Job drawing, mm, ordinate dimensions from the low corner. One solid piece. Round coordinates to 2 decimals unless told otherwise and drop trailing zeros. Loops run counter-clockwise (first coordinate to the right, second up) from the corner with the lowest first, then second, coordinate; pieces in that order, holes last. Notation, with made-up numbers: M 12,-35.75 L 42,-35.75 A33 ccw 42,3.25 Z; hole C 53,-36 d9. An arc over 180 degrees is marked long. Use a Markdown table: item, result. Add a question column.
(1) Band-saw the part on C-C, the plane x = 18. Write the cut outline in (y, z), and give its area (3 significant figures).
(2) Flat gauge pins, fed straight in: P1, Ø1.5, axis at x = 12.5, z = 1.5, coming from the -Y side; P2, Ø6, axis at x = 19, y = 9.5, coming from the -Z side; P3, Ø1.5, axis at y = 15, z = 1, coming from the +X side. Where does each tip first touch, or does it go through?
(3) Band-saw the part on D-D, the plane z = 0.65. Write the cut outline in (x, y) (3 decimals).
(4) Band-saw the part on B-B, the plane x = 11.43. Write the cut outline in (y, z) (3 decimals).
(5) Wall check: L1, parallel to Y at x = 11.43, z = 1.85 (3 decimals); L2, parallel to X at y = 11.75, z = 1.5; L3, parallel to Y at x = 15.25, z = 0.35. Give the ranges that are in metal, low to high.
(6) Band-saw the part on A-A, the plane y = 11.43. Write the cut outline in (x, z) (3 decimals), and give its area (3 significant figures).
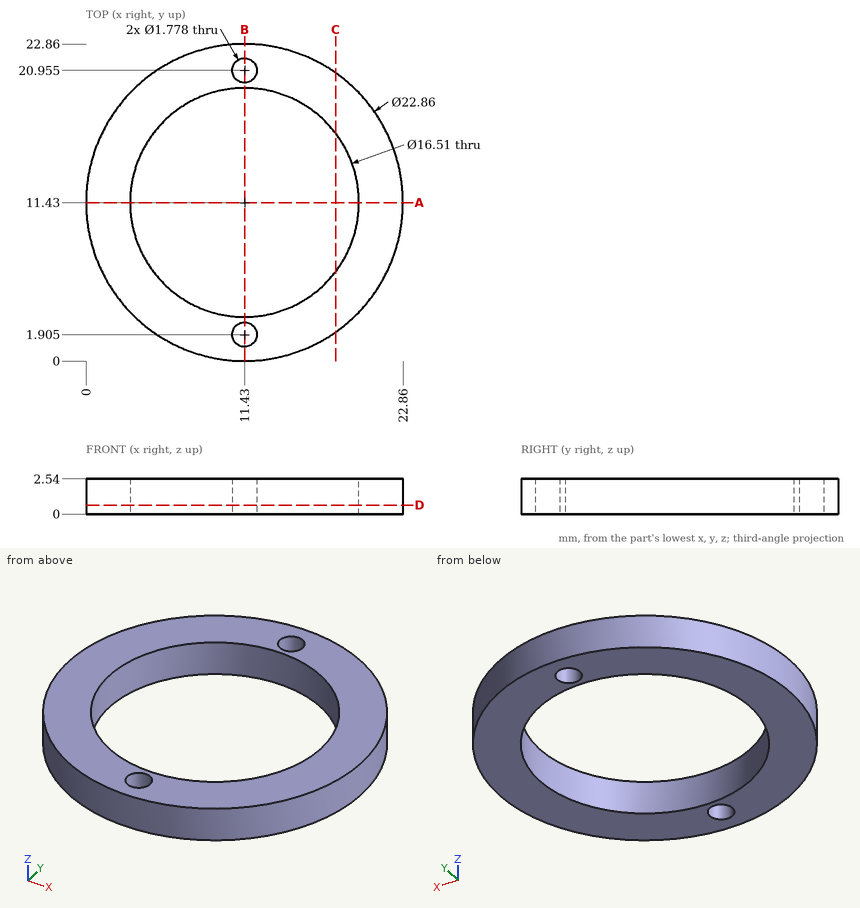
Return value:
| question | item | result |
|---|---|---|
| 1 | outline | M 2.08,0 L 6.43,0 L 6.43,2.54 L 2.08,2.54 Z; M 16.43,0 L 20.78,0 L 20.78,2.54 L 16.43,2.54 Z |
| 1 | area | 22.1 mm^2 |
| 2 | P1 | y = 0 |
| 2 | P2 | z = 0 |
| 2 | P3 | x = 22.51 |
| 3 | outline | C 11.43,11.43 d22.86; hole C 11.43,11.43 d16.51; hole C 11.43,1.905 d1.778; hole C 11.43,20.955 d1.778 |
| 4 | outline | M 0,0 L 1.016,0 L 1.016,2.54 L 0,2.54 Z; M 2.794,0 L 3.175,0 L 3.175,2.54 L 2.794,2.54 Z; M 19.685,0 L 20.066,0 L 20.066,2.54 L 19.685,2.54 Z; M 21.844,0 L 22.86,0 L 22.86,2.54 L 21.844,2.54 Z |
| 5 | L1 | 0 to 1.016, 2.794 to 3.175, 19.685 to 20.066, 21.844 to 22.86 |
| 5 | L2 | 0 to 3.18, 19.68 to 22.86 |
| 5 | L3 | 0.66 to 4.11, 18.75 to 22.2 |
| 6 | outline | M 0,0 L 3.175,0 L 3.175,2.54 L 0,2.54 Z; M 19.685,0 L 22.86,0 L 22.86,2.54 L 19.685,2.54 Z |
| 6 | area | 16.1 mm^2 |
